The model under review builds one solid part; all positions refer to its coordinate system, in mm. Face numbers are marked on the shaded views. A direction names the side the tool comes from. Give positions to 0.01 mm unless a question says otherwise; leave off trailing zeros. Loops run counter-clockwise (first coordinate to the right, second up) from the corner with the lowest first, then second, coordinate; pieces in that order, holes last. Notation, with made-up numbers: M 10.25,76 L 56.25,76 A23 cw 56.25,103 Z; hole C 9.25,47 d5. An arc over 180 degrees is marked long. Return JSON: item names as keys, results as strings. Group by question number.
Autodesk Inventor part; units mm, degrees
ref_plane "YZ Plane" through (0, 0, 0) normal (1, 0, 0) x (0, 1, 0)
ref_plane "XZ Plane" through (0, 0, 0) normal (0, 1, 0) x (-1, 0, 0)
ref_plane "XY Plane" through (0, 0, 0) normal (0, 0, 1) x (1, 0, 0)
sketch "スケッチ1" plane through (0, 0, 0) normal (0, 0, 1) x (1, 0, 0)
  circle A0 centre (0, 0) radius 3.5 construction
  line L0 (3.5, -2.0207) -> (0, -4.0415)
  line L1 (0, -4.0415) -> (-3.5, -2.0207)
  line L2 (-3.5, -2.0207) -> (-3.5, 2.0207)
  line L3 (-3.5, 2.0207) -> (0, 4.0415)
  line L4 (0, 4.0415) -> (3.5, 2.0207)
  line L5 (3.5, 2.0207) -> (3.5, -2.0207)
  point P0 (3.5, 0)
  dimension "d0" = 7
extrude "押し出し1" add sketch "スケッチ1" along normal blind 30
sketch "スケッチ2" plane through (0, 0, 30) normal (0, 0, 1) x (1, 0, 0)
  point P0 (0, 0)
  point P1 (0, 0)
hole "穴1" at (0, 0, 30) direction (0, 0, -1) diameter 4 depth 12 tip angle 118
sketch "スケッチ3" plane through (0, 0, 0) normal (0, 0, -1) x (-1, 0, 0)
  circle A0 centre (0, 0) radius 2
  dimension "d10" = 4
extrude "押し出し2" add sketch "スケッチ3" along normal blind 10
properties part number "六角スペーサー" material "鉄、ダクタイル鋳鉄"
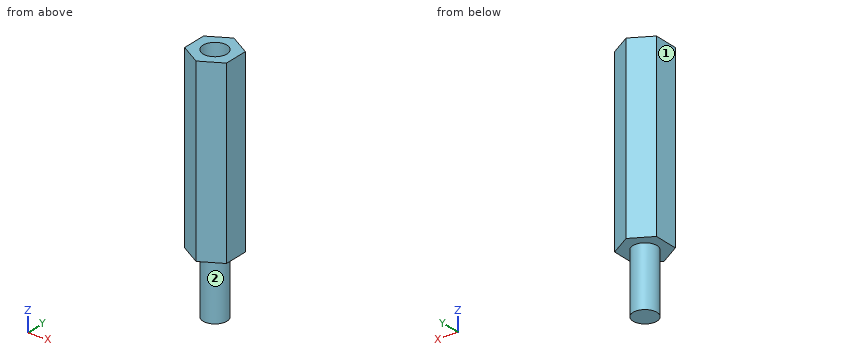
(1) For probe 1 along X at (y, z) = (0, 26.5); probe 2 along Z at (x, y) = (-2, -0.75); probe 3 along Y at (x, z) = (-0.75, 24), list the stretches that pass through material, from the lowest coordinate up.
(2) Add section D-D (x = 3). Write out the cut boundary in (y, z).
(3) For pin 1 (2.5 mm diameter, centred on x = 0, y = 0, fed in from +Z); pin 2 (2 mm diameter, centred on x = -2, y = -3, fed in from -Z); pin 3 (2 mm diameter, centred on x = 0.5, y = -0.5, fed in from +Z), all flat-tipped, find the tip position at first contact; note any pin that passes through.
(4) Add section A-A (z = 26.5). Write out the cut boundary in (x, y).
(5) For the marked faces 1 and 2, list the 3-axis set-ups (+Z, -Z, +X, -X, +Y, -Y) from which the entire face can be reached by the end or side of a thin tool; tool diameter is ignored.
(6) Add section B-B (z = -3). Write out the cut boundary in (x, y), and give its area (3 significant figures).
(7) Add section C-C (y = 2.75). Write out the cut boundary in (x, z), and give its area (3 significant figures).
Verdict:
{
 "1": {"probe 1": "x = -3.5 to -2, 2 to 3.5", "probe 2": "z = 0 to 30", "probe 3": "y = -3.61 to -1.85, 1.85 to 3.61"},
 "2": {"outline": "M -2.31,0 L 2.31,0 L 2.31,30 L -2.31,30 Z"},
 "3": {"pin 1": "stops at z = 17.55", "pin 2": "stops at z = 0", "pin 3": "stops at z = 17.82"},
 "4": {"outline": "M -3.5,-2.02 L 0,-4.04 L 3.5,-2.02 L 3.5,2.02 L 0,4.04 L -3.5,2.02 Z; hole C 0,0 d4"},
 "5": {"face 1": "+Z, -Z, -X, +Y, -Y", "face 2": "-Z"},
 "6": {"outline": "C 0,0 d4", "area": "12.6 mm²"},
 "7": {"outline": "M -2.24,0 L 2.24,0 L 2.24,30 L -2.24,30 Z", "area": "134 mm²"}
}
